from build123d import *

# Parameters (mm, degrees)
MOTOR_SHELL_DEPTH                     = 32.6
MOTOR_MOUNT_DEPTH                     = 4
MOUNTING_HOLE_D                       = 3.4
MOUNTING_HOLE_CSINK_D                 = 6.72
MOUNTING_HOLE_CSINK_ANGLE             = 90
HOLE_DUPLICATION_COUNT                = 3
SKETCH11_R                            = 6.5
SHAFT_BASE_CUTOUT_DEPTH               = 33.6
M3X0_5_TAPPED_HOLE1_D                 = 2.5
M3X0_5_TAPPED_HOLE1_DEPTH             = 10
M3X0_5_TAPPED_HOLE1_CSINK_D           = 3.05
M3X0_5_TAPPED_HOLE1_CSINK_ANGLE       = 90
M3X0_5_TAPPED_HOLE1_TIP               = 0.751075774
M3X0_5_TAPPED_HOLE2_D                 = 2.5
M3X0_5_TAPPED_HOLE2_DEPTH             = 7.5
M3X0_5_TAPPED_HOLE2_CSINK_D           = 3.05
M3X0_5_TAPPED_HOLE2_CSINK_ANGLE       = 90
M3X0_5_TAPPED_HOLE2_TIP               = 0.751075774
M3X0_5_TAPPED_HOLE5_D                 = 2.5
M3X0_5_TAPPED_HOLE5_DEPTH             = 10
M3X0_5_TAPPED_HOLE5_TIP               = 0.751075774
M3X0_5_TAPPED_HOLE6_REACH             = 39
SKETCH26_R                            = 1.35
M3X0_5_TAPPED_HOLE6_DIRECTION_2_REACH = 11
M4X0_7_TAPPED_HOLE1_D                 = 3.3
M4X0_7_TAPPED_HOLE1_DEPTH             = 11.5
M4X0_7_TAPPED_HOLE1_TIP               = 0.991420021
ENLARGE_CAVITY_DEPTH                  = 28.6
MOD_1_DEPTH                           = 28.6
SKETCH31_W                            = 8
SKETCH31_H                            = 7
MOD_2_DEPTH                           = 32.6


with BuildPart() as part:
    # Motor Shell Profile → Motor Shell (new body)
    with BuildSketch(Plane(origin=(0, 0, 0), x_dir=(0, 0, -1), z_dir=(1, 0, 0))):
        with BuildLine():
            Line((25.335548996, 5.840373025), (17, 42))
            Line((17, 42), (17, 50))
            Line((17, 50), (-20, 50))
            Line((-20, 50), (-20, 46))
            Line((-20, 46), (10.895095859, 46))
            ThreePointArc((10.895095859, 46), (12.309309421, 45.414213562), (12.895095859, 44))
            Line((12.895095859, 44), (12.895095859, 42))
            Line((12.895095859, 42), (21.437772227, 4.941854098))
            ThreePointArc((21.437772227, 4.941854098), (17.215121117, -13.69816064), (0, -22))
            Line((0, -22), (-16, -22))
            Line((-16, -22), (-16, -32))
            Line((-16, -32), (13, -32))
            ThreePointArc((13, -32), (15.828427125, -30.828427125), (17, -28))
            Line((17, -28), (17, -21.840329668))
            ThreePointArc((17, -21.840329668), (17.377125597, -19.935327763), (18.451612903, -18.31769585))
            ThreePointArc((18.451612903, -18.31769585), (25.004638765, -7.125169489), (25.335548996, 5.840373025))
        make_face()
    extrude(amount=MOTOR_SHELL_DEPTH)

    # Sketch3 → Motor Mount (add)
    with BuildSketch(Plane(origin=(28.6, 0, 0), x_dir=(0, 0, -1), z_dir=(1, 0, 0))):
        with BuildLine():
            Line((-20, 46), (12.895095859, 46))
            Line((12.895095859, 46), (12.895095859, 42))
            Line((12.895095859, 42), (21.437772227, 4.941854098))
            ThreePointArc((21.437772227, 4.941854098), (17.215121117, -13.69816064), (0, -22))
            Line((0, -22), (-16, -22))
            Line((-16, -22), (-16, 6))
            ThreePointArc((-16, 6), (-16.513167019, 9.16227766), (-18, 12))
            ThreePointArc((-18, 12), (-19.486832981, 14.83772234), (-20, 18))
            Line((-20, 18), (-20, 46))
        make_face()
    extrude(amount=MOTOR_MOUNT_DEPTH)

    # Mounting Hole (through all)
    with Locations(Plane(origin=(32.6, 0, 0), x_dir=(0, 0, -1), z_dir=(1, 0, 0))):
        with Locations((7.070663707, -8.426488874)):
            mounting_hole = CounterSinkHole(MOUNTING_HOLE_D / 2, MOUNTING_HOLE_CSINK_D / 2, counter_sink_angle=MOUNTING_HOLE_CSINK_ANGLE)

    # Hole Duplication: Mounting Hole ×3 about axis
    hole_duplication_axis = Axis((0, 0, 0), (1, 0, 0))
    for i in range(1, HOLE_DUPLICATION_COUNT):
        add(mounting_hole.rotate(hole_duplication_axis, i * 360 / HOLE_DUPLICATION_COUNT), mode=Mode.SUBTRACT)

    # Sketch11 → Shaft Base Cutout (cut, through all)
    with BuildSketch(Plane(origin=(32.6, 0, 0), x_dir=(0, 0, -1), z_dir=(1, 0, 0))):
        Circle(SKETCH11_R)
    extrude(amount=-SHAFT_BASE_CUTOUT_DEPTH, mode=Mode.SUBTRACT)

    # M3x0.5 Tapped Hole1
    with Locations(Plane(origin=(32.6, 0, 0), x_dir=(0, 0, -1), z_dir=(1, 0, 0))):
        with Locations((-8.458892109, -26.736481777), (11.237262951, -23.263518223), (-14.452158477, 18.098247344), (2.289573324, 21.050266364)):
            CounterSinkHole(M3X0_5_TAPPED_HOLE1_D / 2, M3X0_5_TAPPED_HOLE1_CSINK_D / 2, depth=M3X0_5_TAPPED_HOLE1_DEPTH, counter_sink_angle=M3X0_5_TAPPED_HOLE1_CSINK_ANGLE)
            with Locations((0, 0, -(M3X0_5_TAPPED_HOLE1_DEPTH + M3X0_5_TAPPED_HOLE1_TIP / 2))):  # 118° drill point
                Cone(0, M3X0_5_TAPPED_HOLE1_D / 2, M3X0_5_TAPPED_HOLE1_TIP, mode=Mode.SUBTRACT)

    # M3x0.5 Tapped Hole2
    with Locations(Plane(origin=(0, 50, 0), x_dir=(1, 0, 0), z_dir=(0, 1, 0))):
        with Locations((8, 4.5), (8, -11.5), (24, -11.5), (24, 4.5)):
            CounterSinkHole(M3X0_5_TAPPED_HOLE2_D / 2, M3X0_5_TAPPED_HOLE2_CSINK_D / 2, depth=M3X0_5_TAPPED_HOLE2_DEPTH, counter_sink_angle=M3X0_5_TAPPED_HOLE2_CSINK_ANGLE)
            with Locations((0, 0, -(M3X0_5_TAPPED_HOLE2_DEPTH + M3X0_5_TAPPED_HOLE2_TIP / 2))):  # 118° drill point
                Cone(0, M3X0_5_TAPPED_HOLE2_D / 2, M3X0_5_TAPPED_HOLE2_TIP, mode=Mode.SUBTRACT)

    # M3x0.5 Tapped Hole5
    with Locations(Plane.XY.offset(16)):
        with Locations((5, -27), (20, -27)):
            Hole(M3X0_5_TAPPED_HOLE5_D / 2, depth=M3X0_5_TAPPED_HOLE5_DEPTH)
            with Locations((0, 0, -(M3X0_5_TAPPED_HOLE5_DEPTH + M3X0_5_TAPPED_HOLE5_TIP / 2))):  # 118° drill point
                Cone(0, M3X0_5_TAPPED_HOLE5_D / 2, M3X0_5_TAPPED_HOLE5_TIP, mode=Mode.SUBTRACT)

    # Sketch26 → M3x0.5 Tapped Hole6 (cut, up to next)
    with BuildSketch(Plane(origin=(0, 0, -17), x_dir=(-1, 0, 0), z_dir=(0, 0, -1)), mode=Mode.PRIVATE) as m3x0_5_tapped_hole6_sk1:
        with Locations((-10, 25.75)):
            Circle(SKETCH26_R)
    m3x0_5_tapped_hole6_tool1 = extrude(m3x0_5_tapped_hole6_sk1.sketch, amount=-M3X0_5_TAPPED_HOLE6_REACH, mode=Mode.PRIVATE) & part.part
    add(m3x0_5_tapped_hole6_tool1.solids().sort_by_distance((10, 25.75, -17))[0], mode=Mode.SUBTRACT)

    # Sketch26 → M3x0.5 Tapped Hole6 direction 2 (cut, up to next)
    with BuildSketch(Plane(origin=(0, 0, -17), x_dir=(-1, 0, 0), z_dir=(0, 0, -1)), mode=Mode.PRIVATE) as m3x0_5_tapped_hole6_direction_2_sk1:
        with Locations((-10, 25.75)):
            Circle(SKETCH26_R)
    m3x0_5_tapped_hole6_direction_2_tool1 = extrude(m3x0_5_tapped_hole6_direction_2_sk1.sketch, amount=M3X0_5_TAPPED_HOLE6_DIRECTION_2_REACH, mode=Mode.PRIVATE) & part.part
    add(m3x0_5_tapped_hole6_direction_2_tool1.solids().sort_by_distance((10, 25.75, -17))[0], mode=Mode.SUBTRACT)

    # M4x0.7 Tapped Hole1
    with Locations(Plane(origin=(0, -32, 0), x_dir=(-1, 0, 0), z_dir=(0, -1, 0))):
        with Locations((-10, -3)):
            Hole(M4X0_7_TAPPED_HOLE1_D / 2, depth=M4X0_7_TAPPED_HOLE1_DEPTH)
            with Locations((0, 0, -(M4X0_7_TAPPED_HOLE1_DEPTH + M4X0_7_TAPPED_HOLE1_TIP / 2))):  # 118° drill point
                Cone(0, M4X0_7_TAPPED_HOLE1_D / 2, M4X0_7_TAPPED_HOLE1_TIP, mode=Mode.SUBTRACT)

    # Sketch29 → Enlarge Cavity (cut)
    with BuildSketch(Plane.ZY):
        with BuildLine():
            Line((0, -23), (16, -23))
            Line((16, -23), (16, 6))
            ThreePointArc((16, 6), (16.513167019, 9.16227766), (18, 12))
            ThreePointArc((18, 12), (19.486832981, 14.83772234), (20, 18))
            Line((20, 18), (20, 46))
            Line((20, 46), (-11.921321894, 46))
            ThreePointArc((-11.921321894, 46), (-13.335535456, 45.414213562), (-13.921321894, 44))
            Line((-13.921321894, 44), (-13.921321894, 42))
            Line((-13.921321894, 42), (-22.412216419, 5.16648383))
            ThreePointArc((-22.412216419, 5.16648383), (-17.997626623, -14.320804305), (0, -23))
        make_face()
    extrude(amount=-ENLARGE_CAVITY_DEPTH, mode=Mode.SUBTRACT)

    # Sketch30 → Mod 1 (add)
    with BuildSketch(Plane.ZY):
        with BuildLine():
            Line((-16.457051563, 31), (3, 42))
            Line((3, 42), (3, 46))
            Line((3, 46), (-11.921321894, 46))
            ThreePointArc((-11.921321894, 46), (-13.335535456, 45.414213562), (-13.921321894, 44))
            Line((-13.921321894, 44), (-13.921321894, 42))
            Line((-13.921321894, 42), (-16.457051563, 31))
        make_face()
    extrude(amount=-MOD_1_DEPTH)

    # Sketch31 → Mod 2 (cut)
    with BuildSketch(Plane.ZY):
        with Locations((-13, 46.5)):
            Rectangle(SKETCH31_W, SKETCH31_H)
    extrude(amount=-MOD_2_DEPTH, mode=Mode.SUBTRACT)

    # Sketch33 → Hole1 (revolve, cut)
    with BuildSketch(Plane(origin=(17.5, 46.5, -9), x_dir=(0, 1, 0), z_dir=(1, 0, 0))):
        Polygon((0, 0), (0, 3.8), (2.55, 3.8), (2.55, 1.525705169), (2.65, 0), align=None)
    revolve(axis=Axis((17.5, 46.5, -15.445314094), (0, 0, 1)), mode=Mode.SUBTRACT)


solid = part.part
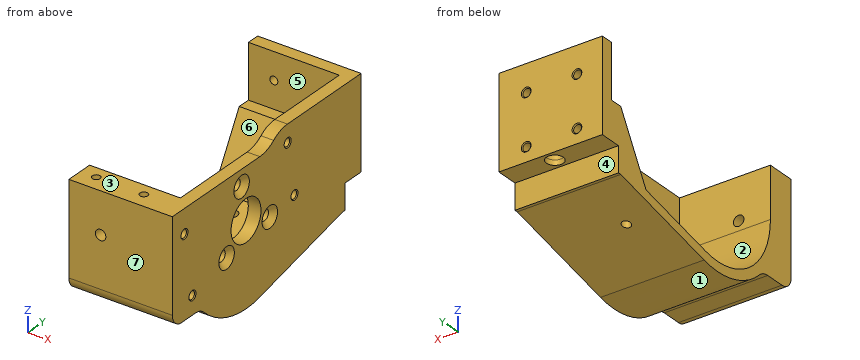
Design review of the part built by this model. Coordinates are the model's own, in mm. Face numbers are marked on the shaded views. A direction names the side the tool comes from. Round coordinates to 2 decimals unless told otherwise and drop trailing zeros. Write each loop counter-clockwise with the first axis right and the second up, starting at its lowest first coordinate (ties: lowest second). Pieces come first, ordered by that corner, then holes. Notation, with made-up numbers: (21.25, 43) - (41.25, 43) arc R17 cw to (41.25, 49) - close; hole circle Ø3 at (-28, 72.25). An arc over 180 degrees is marked (long way). Return JSON: item names as keys, results as strings. Group by question number.
Item 1: For probe 1 along X at (y, z) = (47.55, 11.5); probe 2 along Z at (x, y) = (24, 47.55); probe 3 along Y at (x, z) = (29, 0), list the stretches that pass through material, from the lowest coordinate up. Write a range as [from, to].
Item 2: Insertion check: P1, Ø5.5, axis at y = -1.91, z = 10.83, coming from the +X side; P2, Ø5, axis at x = 20, y = -25, coming from the -Z side; P3, Ø8, axis at x = 20.5, y = -10.5, coming from the -Z side; P4, Ø8, axis at y = 0, z = 0, coming from the -X side. Each pin has a flat end and moves straight along its axis. Give the tip position at first contact, or say it passes through.
Item 3: Machinability: for the marked faces 1, 2 and 3, which of the approach directions +Z, -Z, +X, -X, +Y, -Y give a long, thin tool a straight path to every point of the face, cutting with its end or side? Answer none if there is none.
Item 4: We need section A-A on y = 25.75. Write out the cut boundary in (x, z).
Item 5: We need section B-B on z = 11.5. Give the number of separate pieces and of enclosed holes in the cut face, and give its area (3 significant figures).
Item 6: The part is to be moulded in two halves that separate along Y. For the marked faces 4, 5, 6 and 7, say which applies: pulls with the +Y half, pulls with the -Y half, needs draft (parallel to the pull), parting line crosses it, or undercut.
Model answer:
{
 "1": {"probe 1": "x = [0, 6.75], [9.25, 22.75], [25.25, 32.6]", "probe 2": "z = [-9, -5.75], [-3.25, 10.25], [12.75, 20]", "probe 3": "y = [-32, -6.5], [6.5, 50]"},
 "2": {"P1": "stops at x = 31.99", "P2": "stops at z = -17", "P3": "stops at z = -25.17", "P4": "passes through"},
 "3": {"face 1": "-Z, +X, -X", "face 2": "+Z, -X", "face 3": "+Z, +X, -X, -Y"},
 "4": {"outline": "(0, -20.75) - (8.65, -20.75) - (8.65, -17.67) - (0, -17.67) - close; (11.35, -20.75) - (32.6, -20.75) - (32.6, 20) - (28.6, 20) - (28.6, -17.67) - (11.35, -17.67) - close"},
 "5": {"separate pieces": "4", "enclosed holes": "2", "area": "654 mm²"},
 "6": {"face 4": "pulls with the +Y half", "face 5": "undercut", "face 6": "undercut", "face 7": "pulls with the -Y half"}
}
